```python
from build123d import *

# Parameters (mm, degrees)
SKETCH1_R           = 15
BOSS_EXTRUDE1_DEPTH = 155
BOSS_EXTRUDE2_START = -16
SKETCH2_R           = 15.85
BOSS_EXTRUDE2_DEPTH = 123
SKETCH3_R           = 15
BOSS_EXTRUDE3_DEPTH = 55
SKETCH6_R           = 12.65
CUT_EXTRUDE2_DEPTH  = 212.192909445


with BuildPart() as part:
    # Sketch1 → Boss-Extrude1 (new body)
    with BuildSketch(Plane(origin=(0, 0, 0), x_dir=(1, 0, 0), z_dir=(0, 1, 0))):
        with Locations(Location((0, 0, 0), (0, 0, 270))):
            Circle(SKETCH1_R)
    extrude(amount=BOSS_EXTRUDE1_DEPTH)

    # Sketch2 → Boss-Extrude2 (add)
    with BuildSketch(Plane(origin=(0, 155, 0), x_dir=(1, 0, 0), z_dir=(0, 1, 0)).offset(BOSS_EXTRUDE2_START)):
        with Locations(Location((0, 0, 0), (0, 0, 270))):
            Circle(SKETCH2_R)
    extrude(amount=-BOSS_EXTRUDE2_DEPTH)

    # Sketch3 → Boss-Extrude3 (add)
    with BuildSketch(Plane(origin=(0, 155, 0), x_dir=(1, 0, 0), z_dir=(0, 1, 0))):
        with Locations(Location((0, 0, 0), (0, 0, 270))):
            Circle(SKETCH3_R)
    extrude(amount=BOSS_EXTRUDE3_DEPTH)

    # Sketch6 → Cut-Extrude2 (cut, through all)
    with BuildSketch(Plane.XZ):
        with Locations(Location((0, 0, 0), (0, 0, 270))):
            Circle(SKETCH6_R)
    extrude(amount=-CUT_EXTRUDE2_DEPTH, mode=Mode.SUBTRACT)


solid = part.part
```
Here's how the part is built. I have some questions about the finished solid (model axes, mm). A direction names the side the tool comes from. Coordinates: 2 decimals unless noted, no trailing zeros. Order: outer loops, then holes, each group sorted by start corner. A loop starts at its lowest first (then second) coordinate and runs counter-clockwise, first axis right, second up. Notation, with made-up numbers: (-36.75, 7.25) - (-3.75, 7.25) arc R31 ccw to (-3.75, 33.25) - close; hole circle Ø2 at (32.25, -35). An arc over 180 degrees is marked (long way). One line per question, with ' | ' between items. Start each with the question number.
1. If we section it at A-A (z = 0): Write out the boundary of the cut face in (x, y).
2. Which directions (+Z, -Z, +X, -X, +Y, -Y) give clear straight access to the entire face, cutting with the end or side of a thin tool? Please do faces 1 (the cylindrical face through (0.66, 174.003, -14.985)), 2 (the flat face through (-10, 0, -8)), 3 (the cylindrical face through (0.66, 7.888, -14.985)).
3. If we section it at B-B (x = 0): Write out the boundary of the cut face in (y, z).
4. I'm going to push flat-ended pins straight in: pin 1 Ø8 at (x, y) = (-11.5, 132.5) entering from -Z; pin 2 Ø1.5 at (x, y) = (-2.5, 82.5) entering from -Z; pin 3 Ø3 at (x, z) = (-5.5, 8.5) entering from +Y. Where does each tip first touch, or does it pass through?
5. If we section it at C-C (y = 46.5): Write out the boundary of the cut face in (x, z).
6. Please list where these lines run through material, in increasing order: line 1 along X through (y, z) = (56, 0); line 2 along X through (y, z) = (154.5, 0); line 3 along Z through (x, y) = (5, 46). Write a range as [from, to].
7. If we mould it in two halves opening along X, with no side actions, what happens to faces 4 (the flat face through (-10, 210, -8)), 5 (the cylindrical face through (-9.64, 78.36, -12.58)), 6 (the cylindrical face through (-12.35, 103.53, 2.74))? For each: released by +X, released by -X, zero draft, split by the parting line, or undercut.
Model answer:
1) outline: (-15.85, 16) - (-15, 16) - (-15, 0) - (-12.65, 0) - (-12.65, 210) - (-15, 210) - (-15, 139) - (-15.85, 139) - close; (12.65, 0) - (15, 0) - (15, 16) - (15.85, 16) - (15.85, 139) - (15, 139) - (15, 210) - (12.65, 210) - close
2) face 1: +Y | face 2: +Z, -Z, +X, -X, -Y | face 3: -Y
3) outline: (0, -15) - (16, -15) - (16, -15.85) - (139, -15.85) - (139, -15) - (210, -15) - (210, -12.65) - (0, -12.65) - close; (0, 12.65) - (210, 12.65) - (210, 15) - (139, 15) - (139, 15.85) - (16, 15.85) - (16, 15) - (0, 15) - close
4) pin 1: stops at z = -13.96 | pin 2: stops at z = -15.75 | pin 3: passes through
5) outline: circle Ø31.7 at (0, 0); hole circle Ø25.3 at (0, 0)
6) line 1: x = [-15.85, -12.65], [12.65, 15.85] | line 2: x = [-15, -12.65], [12.65, 15] | line 3: z = [-15.04, -11.62], [11.62, 15.04]
7) face 4: zero draft | face 5: split by the parting line | face 6: undercut
